Geometry check sheet. Reference: the model listing, model coordinates, mm. A direction names the side the tool comes from. Round coordinates to 2 decimals unless told otherwise and drop trailing zeros. Loops run counter-clockwise (first coordinate to the right, second up) from the corner with the lowest first, then second, coordinate; pieces in that order, holes last. Notation, with made-up numbers: M 51,28 L 61,28 A12 ccw 61,49 Z; hole C 0,75 d1. An arc over 180 degrees is marked long. Use one line per item in the form item = value. Start each with the question number.
1. Cross-section at B-B (z = 0). Record the boundary of the cut face in (x, y), then the cut area to 3 significant figures.
2. Material ranges on line 1 (Y direction, x = 4, z = -34); line 2 (Y direction, x = 6.5, z = -1); line 3 (Z direction, x = 9, y = 25.5), recorded low to high.
3. Go/stop test with flat-tipped pins: pin 1 (2 mm diameter, centred on x = 1.5, z = 30, fed in from -Y); pin 2 (4 mm diameter, centred on x = 3.5, z = -19.5, fed in from -Y); pin 3 (3 mm diameter, centred on x = 7.5, z = -6, fed in from +Y). Record where each tip stops, or that it passes through.
4. Cross-section at D-D (y = -20). Record the boundary of the cut face in (x, z).
5. Cross-section at C-C (z = -10). Record the boundary of the cut face in (x, y), then the cut area to 3 significant figures.
6. Draft check along Z on faces 3 (the cylindrical face through (4.82, -5.99, 45.61)), 4 (the cylindrical face through (4.7, -21.4, -36.4)), 5 (the flat face through (9.5, 3, 38)), 6 (the cylindrical face through (5.7, -8.02, -36.12)). Enter one of: pulls with the +Z half, pulls with the -Z half, needs draft (parallel to the pull), parting line crosses it, or undercut.
7. Cross-section at A-A (y = 0). Record the boundary of the cut face in (x, z), then the cut area to 3 significant figures.
8. Set-up check for faces 1 (the flat face through (2, -33.1, -2.6)), 2 (the cylindrical face through (4.68, -17.77, 34.35)): record each of +Z, -Z, +X, -X, +Y, -Y from which the full face is reachable in a straight line by a thin tool's end or side.
```python
from build123d import *

# Parameters (mm, degrees)
ESQUISSE2_R                  = 2.25
ENL_V_MAT_EXTRU_1_DEPTH      = 10.5
R_P_TITION_CIRCULAIRE1_COUNT = 3


with BuildPart() as part:
    # Esquisse1 → Base-Révolution (revolve)
    with BuildSketch(Plane.XY):
        Polygon((0, 33), (0, 46), (9.5, 46), (9.5, 37), (2, 37), (2, 33), align=None)
    revolve(axis=Axis((0, 0, 0), (1, 0, 0)))

    # Esquisse2 → Enlèv. mat.-Extru.1 (cut, through all)
    with BuildSketch(Plane.ZY):
        with Locations((0, 40)):
            Circle(ESQUISSE2_R)
    enl_v_mat_extru_1 = extrude(amount=-ENL_V_MAT_EXTRU_1_DEPTH, mode=Mode.SUBTRACT)

    # Répétition circulaire1: Enlèv. mat.-Extru.1 ×3 about axis
    r_p_tition_circulaire1_axis = Axis((0, 0, 0), (1, 0, 0))
    for i in range(1, R_P_TITION_CIRCULAIRE1_COUNT):
        add(enl_v_mat_extru_1.rotate(r_p_tition_circulaire1_axis, i * 360 / R_P_TITION_CIRCULAIRE1_COUNT), mode=Mode.SUBTRACT)


solid = part.part
```
Reported:
q1.outline = M 0,-46 L 9.5,-46 L 9.5,-37 L 2,-37 L 2,-33 L 0,-33 Z; M 0,33 L 2,33 L 2,37 L 9.5,37 L 9.5,37.75 L 0,37.75 Z; M 0,42.25 L 9.5,42.25 L 9.5,46 L 0,46 Z
q1.area = 144 mm²
q2.line_1 = -30.98 to -22.16, -17.84 to -14.59, 14.59 to 30.98
q2.line_2 = -45.99 to -36.99, 36.99 to 37.98, 42.02 to 45.99
q2.line_3 = -38.29 to -26.81, 26.81 to 38.29
q3.pin_1 = -35.71
q3.pin_2 = -42.54
q3.pin_3 = 45.78
q4.outline = M 0,-41.42 L 9.5,-41.42 L 9.5,-36.89 L 0,-36.89 Z; M 0,-32.39 L 9.5,-32.39 L 9.5,-31.13 L 2,-31.13 L 2,-26.25 L 0,-26.25 Z; M 0,26.25 L 2,26.25 L 2,31.13 L 9.5,31.13 L 9.5,32.39 L 0,32.39 Z; M 0,36.89 L 9.5,36.89 L 9.5,41.42 L 0,41.42 Z
q5.outline = M 0,-44.9 L 9.5,-44.9 L 9.5,-35.62 L 2,-35.62 L 2,-31.45 L 0,-31.45 Z; M 0,31.45 L 2,31.45 L 2,35.62 L 9.5,35.62 L 9.5,44.9 L 0,44.9 Z
q5.area = 193 mm²
q6.face_3 = parting line crosses it
q6.face_4 = undercut
q6.face_5 = needs draft
q6.face_6 = undercut
q7.outline = M 0,-46 L 9.5,-46 L 9.5,-37 L 2,-37 L 2,-33 L 0,-33 Z; M 0,33 L 2,33 L 2,37 L 9.5,37 L 9.5,46 L 0,46 Z
q7.area = 187 mm²
q8.face_1 = +X
q8.face_2 = +X, -X
